Read the model definition and answer for the solid it produces. Units are mm, in the model's axes. Coordinates: 2 decimals unless noted, no trailing zeros. Write each loop counter-clockwise with the first axis right and the second up, starting at its lowest first coordinate (ties: lowest second). Pieces come first, ordered by that corner, then holes. Notation, with made-up numbers: (40.25, 15) - (70.25, 15) arc R13 ccw to (70.25, 28) - close; hole circle Ø8 at (-39.75, 20). An arc over 180 degrees is marked (long way). Use a Markdown table: item, result.
Autodesk Inventor part; units mm, degrees
ref_plane "YZ Plane" through (0, 0, 0) normal (1, 0, 0) x (0, 1, 0)
ref_plane "XZ Plane" through (0, 0, 0) normal (0, 1, 0) x (-1, 0, 0)
ref_plane "XY Plane" through (0, 0, 0) normal (0, 0, 1) x (1, 0, 0)
sketch "スケッチ1" plane through (0, 0, 0) normal (0, 1, 0) x (-1, 0, 0)
  point P0 (0, 0)
sketch "スケッチ2" plane through (0, 0, 0) normal (0, 0, 1) x (1, 0, 0)
  line L0 (0, 0) -> (0, 4)
  line L1 (0, 4) -> (245, 0)
  line L2 (0, 0) -> (245, 0)
  dimension "d0" = 4
  dimension "d1" = 245
extrude "押し出し1" add sketch "スケッチ2" along normal blind 220
sketch "スケッチ4" plane through (0, 0, 220) normal (0, 0, 1) x (1, 0, 0)
  line L0 (0, 4) -> (0, 0)
  line L1 (55, 0) -> (245, 0)
  line L2 (245, 0) -> (245, 4)
  line L3 (245, 4) -> (55, 4)
  line L4 (55, 4) -> (55, 0)
  line L5 (0, 4) -> (45, 4)
  line L6 (45, 4) -> (45, 0)
  line L7 (45, 0) -> (0, 0)
  line L8 (0, 0) -> (0, 4)
  dimension "d8" = 4
  dimension "d9" = 190
  dimension "d10" = 55
  dimension "d23" = 45
extrude "押し出し2" cut sketch "スケッチ4" against normal blind 10
sketch "スケッチ5" plane through (0, 0, 0) normal (0, 0, -1) x (-1, 0, 0)
  line L0 (-55, 0) -> (-245, 0)
  line L1 (-245, 0) -> (-245, 4)
  line L2 (-245, 4) -> (-55, 4)
  line L3 (-55, 4) -> (-55, 0)
  line L4 (0, 4) -> (0, 0)
  line L5 (0, 4) -> (-45, 4)
  line L6 (-45, 4) -> (-45, 0)
  line L7 (-45, 0) -> (0, 0)
  line L8 (0, 0) -> (0, 4)
  dimension "d13" = 4
  dimension "d14" = 55
  dimension "d15" = 190
  dimension "d22" = 45
extrude "押し出し3" cut sketch "スケッチ5" against normal blind 10
sketch "スケッチ6" plane through (0, 0, 0) normal (0, -1, 0) x (1, 0, 0)
  line L0 (0, 0) -> (0, 220)
  line L1 (55, 10) -> (245, 10)
  line L2 (245, 23.5) -> (146, 210)
  line L3 (245, 210) -> (245, 23.5)
  line L4 (146, 210) -> (245, 23.5)
  line L5 (146, 210) -> (245, 210)
  line L6 (245, 210) -> (55, 210)
  dimension "d18" = 146
  dimension "d19" = 13.5
extrude "押し出し4" cut sketch "スケッチ6" against normal blind 10
properties part number "坂"
(1) A cutting plane is placed at D-D, the plane z = 185. Write down the section's boundary in (x, y), and give its area (3 significant figures).
Report:
| item | result |
|---|---|
| outline | (0, 0) - (159.27, 0) - (159.27, 1.4) - (0, 4) - close |
| area | 430 mm² |
(2) Straight lines are drawn through the part: L1, parallel to Z at x = 13.5, y = 3.35; L2, parallel to Y at x = 147, z = 61.5; L3, parallel to Y at x = 51, z = 48. For each, find the intervals that lie inside material, in ascending order.
Report:
| item | result |
|---|---|
| L1 | z = 10 to 210 |
| L2 | y = 0 to 1.6 |
| L3 | y = 0 to 3.17 |
(3) A cutting plane is placed at A-A, the plane y = 2.3. Write down the section's boundary in (x, z) (3 decimals).
Report:
| item | result |
|---|---|
| outline | (0, 10) - (45, 10) - (45, 0) - (55, 0) - (55, 10) - (104.125, 10) - (104.125, 210) - (55, 210) - (55, 220) - (45, 220) - (45, 210) - (0, 210) - close |
(4) Each of these flat-tipped pins is pushed along its axis until it touches: P1, Ø2, axis at y = 1.5, z = 168.5, coming from the +X side; P2, Ø1.6, axis at y = 1.5, z = 214.5, coming from the +X side; P3, Ø10, axis at x = 167.5, z = 153.5, coming from the +Y side; P4, Ø3, axis at x = 39, z = 34, coming from the -Y side. Where does it stop, or does it pass through?
Report:
| item | result |
|---|---|
| P1 | stops at x = 168.54 |
| P2 | stops at x = 55 |
| P3 | stops at y = 1.35 |
| P4 | stops at y = 0 |
(5) A cutting plane is placed at C-C, the plane x = 202. Write down the section's boundary in (y, z), and give its area (3 significant figures).
Report:
| item | result |
|---|---|
| outline | (0, 10) - (0.7, 10) - (0.7, 104.51) - (0, 104.51) - close |
| area | 66.3 mm² |
(6) A cutting plane is placed at B-B, the plane z = 14.5. Write down the section's boundary in (x, y), and give its area (3 significant figures).
Report:
| item | result |
|---|---|
| outline | (0, 0) - (245, 0) - (0, 4) - close |
| area | 490 mm² |
